Check sheet for the modelled part. Datum: model origin and axes. Units: mm. Face numbers are marked on the shaded views. Round coordinates to 2 decimals unless told otherwise and drop trailing zeros. Write each loop counter-clockwise with the first axis right and the second up, starting at its lowest first coordinate (ties: lowest second). Pieces come first, ordered by that corner, then holes.
Item 1: Release check for a two-part mould opening along Y. For the marked faces 1, 2 and 3 record: +Y half, -Y half, draft (parallel to the pull), parting line (faces both ways), or undercut.
Item 2: Material ranges on line 1 (Y direction, x = -1, z = 5.2); line 2 (Y direction, x = 1.5, z = 1.3); line 3 (X direction, y = 1, z = 3.4), recorded low to high.
Item 3: Cross-section at D-D on y = 4.5. Enter the section's corners in (x, z).
Item 4: Cross-section at A-A on z = 5.05. Enter the section's corners in (x, y).
Item 5: Go/stop test with flat-tipped pins: pin 1 Ø3 at (x, z) = (-2.5, 2.5) entering from +Y; pin 2 Ø1.6 at (y, z) = (-6.5, 3.5) entering from +X. Record where each tip stops, or that it passes through.
Item 6: Cross-section at C-C on x = 1. Enter the section's corners in (y, z).
Item 7: Cross-section at B-B on y = -0.5. Enter the section's corners in (x, z).
from build123d import *

# Parameters (mm, degrees)
F0_R     = 1.7
F1_DEPTH = 5.5


with BuildPart() as f1:
    # F0 (on Top) → F1 (new body)
    with BuildSketch(Plane.XY):
        with BuildLine():
            ThreePointArc((-3.024665, 2.461991), (0.769594, 3.823313), (3.741657, 1.1))
            ThreePointArc((3.741657, 1.1), (1.866017, 11.083336), (-3, 20))
            ThreePointArc((-3, 20), (-1.70213, 11.229153), (-3.024665, 2.461991))
        make_face()
        with BuildLine():
            ThreePointArc((2.714774, -2.8), (3.591491, -1.52026), (3.9, 0))
            ThreePointArc((3.9, 0), (3.860211, 0.555669), (3.741657, 1.1))
            ThreePointArc((3.741657, 1.1), (0.769594, 3.823313), (-3.024665, 2.461991))
            ThreePointArc((-3.024665, 2.461991), (-3.435515, 1.221461), (-3.9, 0))
            ThreePointArc((-3.9, 0), (-3.759503, -1.037371), (-3.348134, -2))
            ThreePointArc((-3.348134, -2), (-0.510182, -3.866486), (2.714774, -2.8))
        make_face()
        Circle(F0_R, mode=Mode.SUBTRACT)
        with BuildLine():
            Line((2.714774, -8.741404), (2.714774, -2.8))
            ThreePointArc((2.714774, -2.8), (-0.510182, -3.866486), (-3.348134, -2))
            Line((-3.348134, -2), (-1.2, -16.845387))
            Line((-1.2, -16.845387), (2.714774, -8.741404))
        make_face()
    extrude(amount=F1_DEPTH)


solid = f1.part
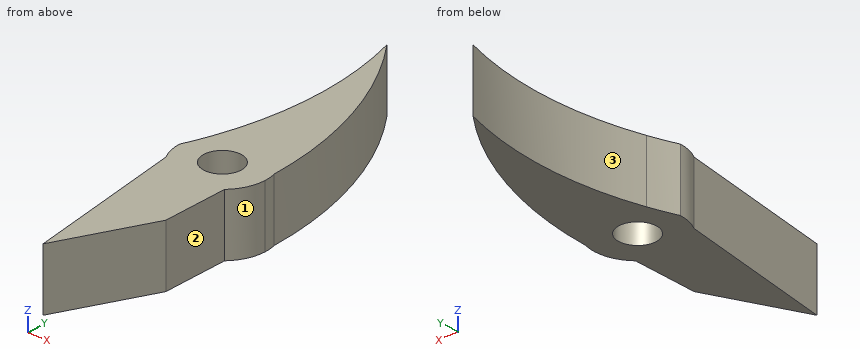
Response values:
1. face 1: -Y half
1. face 2: draft
1. face 3: undercut
2. line 1: y = -16.43 to -1.37, 1.37 to 17.09
2. line 2: y = -11.26 to -0.8, 0.8 to 12.06
2. line 3: x = -3.52 to -1.37, 1.37 to 3.77
3. outline: (-2.48, 0) - (3.46, 0) - (3.46, 5.5) - (-2.48, 5.5) - close
4. outline: (-3.9, 0) arc R3.9 ccw to (-3.35, -2) - (-1.2, -16.85) - (2.71, -8.74) - (2.71, -2.8) arc R3.9 ccw to (3.9, 0) arc R3.9 ccw to (3.74, 1.1) arc R32.5 ccw to (-3, 20) arc R30 cw to (-3.02, 2.46) arc R30 cw to start; hole circle Ø3.4 at (0, 0)
5. pin 1: stops at y = 20
5. pin 2: stops at x = 2.71
6. outline: (-12.29, 0) - (-1.37, 0) - (-1.37, 5.5) - (-12.29, 5.5) - close; (1.37, 0) - (13.26, 0) - (13.26, 5.5) - (1.37, 5.5) - close
7. outline: (-3.87, 0) - (-1.62, 0) - (-1.62, 5.5) - (-3.87, 5.5) - close; (1.62, 0) - (3.87, 0) - (3.87, 5.5) - (1.62, 5.5) - close
